Geometry: final body of the model. Coordinates: model frame, mm. Face numbers are marked on the shaded views. A direction names the side the tool comes from. Coordinates: 2 decimals unless noted, no trailing zeros. Order: outer loops, then holes, each group sorted by start corner. A loop starts at its lowest first (then second) coordinate and runs counter-clockwise, first axis right, second up. Notation, with made-up numbers: (3, -0.5) -> (7, -0.5) arc R10 cw to (7, 17.5) -> close; hole circle Ø6 at (-28.75, 27). An arc over 180 degrees is marked (long way). Use one line per item in the form item = value.
Autodesk Inventor part; units mm, degrees
ref_plane "YZ Plane" through (0, 0, 0) normal (1, 0, 0) x (0, 1, 0)
ref_plane "XZ Plane" through (0, 0, 0) normal (0, 1, 0) x (-1, 0, 0)
ref_plane "XY Plane" through (0, 0, 0) normal (0, 0, 1) x (1, 0, 0)
sketch "Boceto1" plane through (0, 0, 0) normal (0, 0, 1) x (1, 0, 0)
  line L0 (-20, 20) -> (20, 20)
  line L1 (20, 20) -> (20, -20)
  line L2 (20, -20) -> (-20, -20)
  line L3 (-20, -20) -> (-20, 20)
  line L4 (-20, 20) -> (20, -20) construction
  line L5 (-18, 18) -> (18, 18)
  line L6 (18, 18) -> (18, -18)
  line L7 (18, -18) -> (-18, -18)
  line L8 (-18, -18) -> (-18, 18)
  line L9 (-18, 0) -> (-20, 0) construction
  line L10 (0, 18) -> (0, 20) construction
  line L11 (18, 0) -> (20, 0) construction
  line L12 (0, -18) -> (0, -20) construction
  point P0 (0, 0)
  point P1 (0, 0)
  dimension "d0" = 40
  dimension "d1" = 2
extrude "Extrusión1" add sketch "Boceto1" along normal blind 370
properties part number "C_358_40_2"
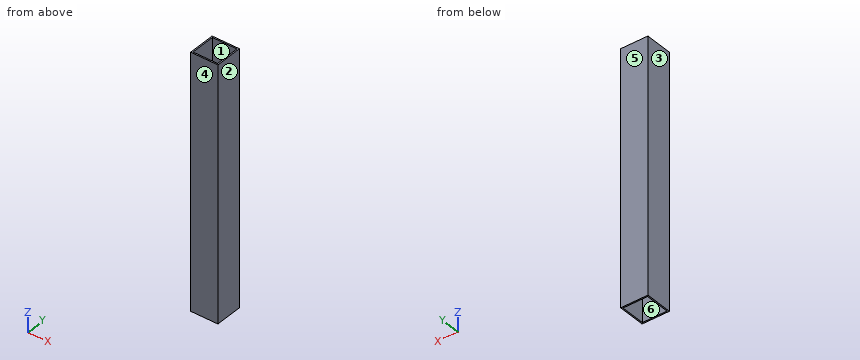
1) Access query for the marked faces 5 and 6. Directions: +Z, -Z, +X, -X, +Y, -Y. A direction counts if a zero-diameter tool reaches every point of the face in a straight line with its end or side. Return the directions, or none.
Results found:
face_5 = +Z, -Z, +X, -X, +Y
face_6 = +Z, -Z
2) Pull-direction query (X, two-part tool) for the marked faces 1, 2, 3 and 4; classes: released by +X, released by -X, zero draft, split by the parting line, or undercut.
Results found:
face_1 = undercut
face_2 = released by +X
face_3 = released by -X
face_4 = zero draft
3) Material intervals for probe 1 along Y at (x, z) = (-8, 120), sorted ascending. Write a range as from..to.
Results found:
probe_1 = -20..-18, 18..20
4) Section A-A, the plane x = 12. Output: boundary loops of the cut face in (y, z), and give its area (3 significant figures).
Results found:
outline = (-20, 0) -> (-18, 0) -> (-18, 370) -> (-20, 370) -> close; (18, 0) -> (20, 0) -> (20, 370) -> (18, 370) -> close
area = 1,480 mm2
5) Section C-C, the plane z = 237. Output: boundary loops of the cut face in (x, y), and give its area (3 significant figures).
Results found:
outline = (-20, -20) -> (20, -20) -> (20, 20) -> (-20, 20) -> close; hole (-18, -18) -> (18, -18) -> (18, 18) -> (-18, 18) -> close
area = 304 mm2
